Part model, mm, in its own coordinate system. A direction names the side the tool comes from. Round coordinates to 2 decimals unless told otherwise and drop trailing zeros. Write each loop counter-clockwise with the first axis right and the second up, starting at its lowest first coordinate (ties: lowest second). Pieces come first, ordered by that corner, then holes. Notation, with made-up numbers: M 14,86.25 L 25,86.25 A35 ccw 25,122.25 Z; hole C 54.25,65 d6. An arc over 180 degrees is marked long. Answer as a JSON object with one key per item and string values. Group by question number.
1. Drop flat-ended pins along their axis: pin 1 (1.5 mm diameter, centred on x = 3.5, z = 0.5, fed in from +Y); pin 2 (4 mm diameter, centred on y = 2.5, z = 4, fed in from -X); pin 3 (2 mm diameter, centred on x = 1, z = 3.5, fed in from -Y); pin 4 (1.5 mm diameter, centred on y = 12, z = 0.5, fed in from +X). Give the stop position or say it passes through.
2. Band-saw the part on B-B, the plane x = 0. Write the cut outline in (y, z).
3. Band-saw the part on D-D, the plane y = 9.75. Write the cut outline in (x, z).
4. Band-saw the part on A-A, the plane z = 0. Write the cut outline in (x, y).
5. Band-saw the part on C-C, the plane y = 15.5. Write the cut outline in (x, z), plus the area to 3 significant figures.
6. Which spindle directions (+Z, -Z, +X, -X, +Y, -Y) get a long thin tool onto all of the face, cutting with end or side? Do faces 1 (the face through (2, 11.112, -2)), 2 (the face through (0, 0, 0)). Say none if no direction does.
7. Drill centre lines: line 1 (Z direction, x = 0, y = 15); line 2 (Y direction, x = -3.25, z = 2.75). Where is each one in solid material? Low to high. Write a range as from..to.
from build123d import *

# Parameters (mm, degrees)
SKETCH1_R           = 5.55625
BOSS_EXTRUDE1_DEPTH = 1.5875
SKETCH2_R           = 3.96875
BOSS_EXTRUDE2_DEPTH = 9.525
SKETCH3_R           = 2.38125
SKETCH3_R_2         = 0.79375
EXTRUDE_THIN2_DEPTH = 7.9248
FILLET1_R           = 0.254


with BuildPart() as part:
    # Sketch1 → Boss-Extrude1 (new body)
    with BuildSketch(Plane(origin=(0, 0, 0), x_dir=(1, 0, 0), z_dir=(0, 1, 0))):
        with Locations(Location((0, 0, 0), (0, 0, 270))):
            Circle(SKETCH1_R)
    extrude(amount=BOSS_EXTRUDE1_DEPTH)

    # Sketch2 → Boss-Extrude2 (add)
    with BuildSketch(Plane(origin=(0, 1.5875, 0), x_dir=(1, 0, 0), z_dir=(0, 1, 0))):
        with Locations(Location((0, 0, 0), (0, 0, 90))):
            Circle(SKETCH2_R)
    extrude(amount=BOSS_EXTRUDE2_DEPTH)

    # Sketch3 → Extrude-Thin2 (add)
    with BuildSketch(Plane(origin=(0, 11.1125, 0), x_dir=(1, 0, 0), z_dir=(0, 1, 0))):
        Circle(SKETCH3_R)
        Circle(SKETCH3_R_2, mode=Mode.SUBTRACT)
    extrude(amount=EXTRUDE_THIN2_DEPTH)

    # Fillet1
    fillet1_edges = [part.edges().sort_by_distance(p)[0] for p in [
        (0, 0, -5.55625),
    ]]
    fillet(fillet1_edges, radius=FILLET1_R)


solid = part.part
Worked answers:
{
 "1": {"pin 1": "stops at y = 11.11", "pin 2": "stops at x = -5.09", "pin 3": "stops at y = 0", "pin 4": "stops at x = 2.38"},
 "2": {"outline": "M 0,-5.3 A0.25 ccw 0.25,-5.56 L 1.59,-5.56 L 1.59,-3.97 L 11.11,-3.97 L 11.11,-2.38 L 19.04,-2.38 L 19.04,-0.79 L 11.11,-0.79 L 11.11,0.79 L 19.04,0.79 L 19.04,2.38 L 11.11,2.38 L 11.11,3.97 L 1.59,3.97 L 1.59,5.56 L 0.25,5.56 A0.25 ccw 0,5.3 Z"},
 "3": {"outline": "C 0,0 d7.94"},
 "4": {"outline": "M -5.56,0.25 A0.25 ccw -5.3,0 L 5.3,0 A0.25 ccw 5.56,0.25 L 5.56,1.59 L 3.97,1.59 L 3.97,11.11 L 2.38,11.11 L 2.38,19.04 L 0.79,19.04 L 0.79,11.11 L -0.79,11.11 L -0.79,19.04 L -2.38,19.04 L -2.38,11.11 L -3.97,11.11 L -3.97,1.59 L -5.56,1.59 Z"},
 "5": {"outline": "C 0,0 d4.76; hole C 0,0 d1.59", "area": "15.8 mm^2"},
 "6": {"face 1": "+Y", "face 2": "+Z, -Z, +X, -X, -Y"},
 "7": {"line 1": "z = -2.38..-0.79, 0.79..2.38", "line 2": "y = 0..1.59"}
}
